from build123d import *

# Parameters (mm, degrees)
F0_W     = 36
F0_H     = 56
F1_DEPTH = 15
F3_DEPTH = 28
F4_D     = 5.5
F5_DEPTH = 15


with BuildPart() as f1:
    # F0 (on Top) → F1 (new body)
    with BuildSketch(Plane.XY):
        Rectangle(F0_W, F0_H)
    extrude(amount=F1_DEPTH)

    # F2 (on Front) → F3 (join)
    with BuildSketch(Plane.XZ):
        Polygon((-17.9443880916, 0), (-18, 15), (-41.1238394028, 30.7888584537), (-41.1238394028, 25.5634840578), (-28.7360682942, 17.105167029), (-28.7360682942, 13.1013058126), (-41.1238394028, 21.5596228414), (-41.1238394028, 15.7888584537), align=None)
        Polygon((28.7360682942, 17.105167029), (41.1238394028, 25.5634840578), (41.1238394028, 30.7888584537), (18, 15), (17.9443880916, 0), (41.1238394028, 15.7888584537), (41.1238394028, 21.5596228414), (28.7360682942, 13.1013058126), align=None)
    extrude(amount=F3_DEPTH)

    # F4 (through all)
    with Locations(Plane(origin=(0, 0, 0), x_dir=(1, 0, 0), z_dir=(0, 0, -1))):
        with Locations((-10, 20), (10, 20), (10, -20), (-10, -20)):
            Hole(F4_D / 2)

    # F5 (add): a face of the model
    f5_faces = [f1.faces().sort_by_distance(p)[0] for p in [
        (0, 0, 15),
    ]]
    extrude(f5_faces, amount=F5_DEPTH)


solid = f1.part
For this review, take the finished solid that the model builds, in its own axes (mm). A direction names the side the tool comes from. Round coordinates to 2 decimals unless told otherwise and drop trailing zeros. Loops run counter-clockwise (first coordinate to the right, second up) from the corner with the lowest first, then second, coordinate; pieces in that order, holes last. Notation, with made-up numbers: (63, -5) - (109, -5) arc R12 cw to (109, 17) - close; hole circle Ø3 at (-21.5, -35.75). An arc over 180 degrees is marked (long way). Use one line per item in the form item = value.
Item 1: Consider section C-C on z = 19. State how many separate pieces and enclosed holes the cut face has, then the cut area to 3 significant figures.
Answers:
separate_pieces = 5
enclosed_holes = 4
area = 2,560 mm^2
Item 2: For line 1 (Y direction, x = -10, z = 18.25); line 2 (X direction, y = 20, z = 6.75); line 3 (X direction, y = -20, z = 8.75), list the stretches that pass through material, from the lowest coordinate up.
Answers:
line_1 = -28 to -22.75, -17.25 to 17.25, 22.75 to 28
line_2 = -18 to -12.75, -7.25 to 7.25, 12.75 to 18
line_3 = -30.79 to -12.75, -7.25 to 7.25, 12.75 to 30.79
Item 3: Tool access review of faces 1 (the flat face through (34.843, -13.804, 21.275)), 2 (the flat face through (-29.4, -13.804, 22.784)), 3 (the flat face through (29.4, -13.804, 7.803)): name each direction out of +Z, -Z, +X, -X, +Y, -Y from which nothing blocks a thin tool from reaching the whole face with its end or side.
Answers:
face_1 = +Y, -Y
face_2 = +Z, +Y, -Y
face_3 = -Z, +X, +Y, -Y
Item 4: Consider section A-A on y = 20. Write out the cut boundary in (x, z), then the cut area to 3 significant figures.
Answers:
outline = (-18, 0) - (-12.75, 0) - (-12.75, 30) - (-18, 30) - close; (-7.25, 0) - (7.25, 0) - (7.25, 30) - (-7.25, 30) - close; (12.75, 0) - (18, 0) - (18, 30) - (12.75, 30) - close
area = 750 mm^2
Item 5: Mouldability with a two-part tool opening along X and no side actions: class faces 4 (the flat face through (29.72, -13.8, 23)), 5 (the flat face through (-27, 0, 16)), 6 (the flat face through (-29.72, -13.8, 8.02)) as +X half, -X half, draft (parallel to the pull), parting line (faces both ways), or undercut.
Answers:
face_4 = undercut
face_5 = draft
face_6 = -X half
Item 6: Clearance check with flat-ended pins moving along their axes: P1, Ø11, axis at x = 1, y = -8, coming from the +Z side; P2, Ø1, axis at y = 12.5, z = 16.5, coming from the -X side; P3, Ø3, axis at x = -32, y = -1, coming from the -Z side. State where each tip first meets the part, or that it passes through.
Answers:
P1 = 30
P2 = -18
P3 = 8.55
Item 7: Consider section B-B on x = -10. Write out the cut boundary in (y, z).
Answers:
outline = (-28, 0) - (-22.75, 0) - (-22.75, 30) - (-28, 30) - close; (-17.25, 0) - (17.25, 0) - (17.25, 30) - (-17.25, 30) - close; (22.75, 0) - (28, 0) - (28, 30) - (22.75, 30) - close
Item 8: Consider section D-D on z = 6. Write out the cut boundary in (x, y), then the cut area to 3 significant figures.
Answers:
outline = (-26.75, -28) - (26.75, -28) - (26.75, 0) - (18, 0) - (18, 28) - (-18, 28) - (-18, 0) - (-26.75, 0) - close; hole circle Ø5.5 at (-10, -20); hole circle Ø5.5 at (-10, 20); hole circle Ø5.5 at (10, -20); hole circle Ø5.5 at (10, 20)
area = 2,410 mm^2
